For this review, take the finished solid that the model builds, in its own axes (mm). A direction names the side the tool comes from. Give positions to 0.01 mm unless a question says otherwise; leave off trailing zeros. Loops run counter-clockwise (first coordinate to the right, second up) from the corner with the lowest first, then second, coordinate; pieces in that order, holes last. Notation, with made-up numbers: (22.25, 61) - (38.25, 61) arc R22 ccw to (38.25, 93) - close; hole circle Ø9 at (-39, -38.75). An arc over 180 degrees is marked (long way). Put each result on its own line as item: value.
Autodesk Inventor part; units mm, degrees
ref_plane "YZ Plane" through (0, 0, 0) normal (1, 0, 0) x (0, 1, 0)
ref_plane "XZ Plane" through (0, 0, 0) normal (0, 1, 0) x (-1, 0, 0)
ref_plane "XY Plane" through (0, 0, 0) normal (0, 0, 1) x (1, 0, 0)
sketch "Sketch1" plane through (0, 0, 0) normal (0, 1, 0) x (-1, 0, 0)
  arc A0 (7.5, 0) -> (-7.5, 0) centre (0, 0) ccw
  arc A1 (2.4, 0) -> (-2.4, 0) centre (0, 0) ccw
  line L0 (-7.5, 0) -> (7.5, 0) construction
  line L1 (0, 0) -> (0, 11.6178) construction
  line L2 (-7.5, 0) -> (-7.5, -7.5)
  line L3 (-2.4, 0) -> (-2.4, -7.5)
  line L4 (2.4, 0) -> (2.4, -7.5)
  line L5 (7.5, 0) -> (7.5, -7.5)
  line L6 (-7.5, -7.5) -> (-2.4, -7.5)
  line L7 (2.4, -7.5) -> (7.5, -7.5)
  dimension "d0" = 15
  dimension "d2" = 7.5
  dimension "d3" = 4.8
  dimension "d6" = 7.5
  dimension "d8" = 7.5
extrude "Extrusion1" add sketch "Sketch1" against normal blind 3
sketch "Sketch2" plane through (0, -3, 0) normal (0, -1, 0) x (1, 0, 0)
  arc A0 (7.5, 0) -> (-7.5, 0) centre (0, 0) ccw
  line L0 (-7.5, 0) -> (-7.5, -7.5)
  line L1 (-2.4, -7.5) -> (-2.4, 0)
  arc A1 (2.4, 0) -> (-2.4, 0) centre (0, 0) ccw
  line L2 (2.4, 0) -> (2.4, -7.5)
  line L3 (7.5, -7.5) -> (7.5, 0)
  arc A2 (2.4, -5.4991) -> (-2.4, -5.4991) centre (0, 0) ccw
  arc A3 (7.5, 0) -> (-7.5, 0) centre (0, 0) ccw
  line L4 (-7.5, 0) -> (-7.5, -7.5)
  line L5 (-2.4, -7.5) -> (-2.4, -5.4991)
  line L6 (2.4, -5.4991) -> (2.4, -7.5)
  line L7 (7.5, -7.5) -> (7.5, 0)
  line L8 (-7.5, -7.5) -> (-2.4, -7.5)
  line L9 (2.4, -7.5) -> (7.5, -7.5)
  dimension "d11" = 6
extrude "Extrusion2" add sketch "Sketch2" along normal blind 3 contours L3 L9 L2 A2 L1 L8 L0 A0
fillet "Fillet1" radius 1.2 1 edges at (7.5, -3, -7.5)
fillet "Fillet2" radius 1.2 3 edges at (2.4, -3, -7.5) (-2.4, -3, -7.5) (-7.5, -3, -7.5)
sketch "Sketch3" plane through (0, -3, 0) normal (0, -1, 0) x (1, 0, 0)
  arc A0 (2.4, -5.4991) -> (-2.4, -5.4991) centre (0, 0) ccw
  line L0 (-2.4, -5.4991) -> (-2.4, 0)
  arc A1 (2.4, 0) -> (-2.4, 0) centre (0, 0) ccw
  line L1 (2.4, 0) -> (2.4, -5.4991)
  line L2 (0, 13.9059) -> (0, -15.9339) construction
  line L3 (-15.9969, 0.3837) -> (17.7517, -5.5671) construction
  line L4 (-15.1634, 5.1107) -> (18.5852, -0.84) construction
  line L5 (-2.4, -15.573) -> (-2.4, 20.0388) construction
  line L6 (2.4, -5.4991) -> (2.4, -2.8602)
  line L7 (4.9988, -3.3184) -> (2.4, -2.8602)
  line L8 (-4.9988, 3.3184) -> (-2.4, 2.8602)
  line L9 (-2.4, 5.4991) -> (-2.4, 2.8602)
  arc A2 (-3, 5.1962) -> (-4.9988, 3.3184) centre (0, 0) ccw
  arc A3 (2.4, -5.4991) -> (4.9988, -3.3184) centre (0, 0) ccw
  dimension "d27" = 80
extrude "Extrusion3" add sketch "Sketch3" along normal blind 3 contours L1 L7 A0 | L9 L8 A0
equation "\"d0\" = HeadConnectorOuterSize"
equation "\"d2\" = 0.5 * HeadConnectorOuterSize"
equation "\"d3\" = HeadConnectorWidth"
equation "\"d6\" = 0.5 * HeadConnectorOuterSize"
equation "\"d8\" = 0.5 * HeadConnectorOuterSize"
equation "\"d9\" = HeadConnectorOuterHeight"
equation "\"d11\" = 0.5 * HeadConnectorDiam"
equation "\"d12\" = HeadConnectorHeight"
equation "\"d14\" = 0.2 * HeadConnectorProportion"
equation "\"d15\" = 0.2 * HeadConnectorProportion"
equation "\"d28\" = HeadConnectorHeight"
equation "\"HeadConnectorDiam\" = 2 * HeadConnectorProportion"
equation "\"HeadConnectorWidth\" = 0.8 * HeadConnectorProportion"
equation "\"HeadConnectorOuterSize\" = 2.5 * HeadConnectorProportion"
equation "\"HeadConnectorHeight\" = 0.5 * HeadConnectorProportion"
equation "\"HeadConnectorOuterHeight\" = 0.5 * HeadConnectorProportion"
equation "\"HeadConnectorTolerance\" = 0.2"
equation "\"HeadConnectorProportion\" = 0.6"
properties part number "HeadConnector"
1) For faces 1 (the face through (-2.4, -4, 4)), 2 (the face through (-7.158, -3.042, -7.139)), 3 (the face through (-2.761, -3.042, -7.158)), 4 (the face through (-3.718, -4.479, 3.093)), 5 (the face through (5, -3, -7.5)), list the 3-axis set-ups (+Z, -Z, +X, -X, +Y, -Y) from which the entire face can be reached by the end or side of a thin tool; tool diameter is ignored.
Geometry check:
face 1: -Z, -Y
face 2: -Z, -X, +Y, -Y
face 3: -Z, +Y, -Y
face 4: -Y
face 5: -Z, +X, -X, +Y, -Y
2) Insertion check: pin 1 Ø1.5 at (x, y) = (1, -2) entering from +Z; pin 2 Ø1.5 at (x, y) = (3.5, -3) entering from +Z; pin 3 Ø3 at (y, z) = (-5, 4) entering from +X. Each pin has a flat end and moves straight along its axis. Give the tip position at first contact, or say it passes through.
Geometry check:
pin 1: stops at z = 7.5
pin 2: stops at z = 6.98
pin 3: stops at x = 7.07
3) Take a section at A-A on z = -2. State the section outline as (x, y) points.
Geometry check:
outline: (-7.5, -6) - (-5.66, -6) - (-5.66, -3) - (-2.4, -3) - (-2.4, 0) - (-7.5, 0) - close; (2.4, -3) - (5.66, -3) - (5.66, -6) - (7.5, -6) - (7.5, 0) - (2.4, 0) - close
4) Take a section at C-C on y = -2.65. State the section outline as (x, z) points.
Geometry check:
outline: (-7.5, -6.3) arc R1.2 ccw to (-6.3, -7.5) - (-3.6, -7.5) arc R1.2 ccw to (-2.4, -6.3) - (-2.4, 0) arc R2.4 cw to (2.4, 0) - (2.4, -6.3) arc R1.2 ccw to (3.6, -7.5) - (6.3, -7.5) arc R1.2 ccw to (7.5, -6.3) - (7.5, 0) arc R7.5 ccw to (-7.5, 0) - close
5) Take a section at D-D on z = 4.25. State the section outline as (x, y) points.
Geometry check:
outline: (-6.18, -6) - (-2.4, -6) - (-2.4, -3) - (4.24, -3) - (4.24, -6) - (6.18, -6) - (6.18, 0) - (-6.18, 0) - close
6) Draft analysis for pull direction X (two halves, no side actions). For faces 6 (the face through (0, -3, 3)), 7 (the face through (-7.5, -3, -3)), 8 (the face through (2, 0, 2)), state which applies: pulls with the +X half, pulls with the -X half, needs draft (parallel to the pull), parting line crosses it, or undercut.
Geometry check:
face 6: undercut
face 7: pulls with the -X half
face 8: needs draft
7) Take a section at B-B on x = 0. State the section outline as (y, z) points, and give its area (3 significant figures).
Geometry check:
outline: (-6, 6) - (-3, 6) - (-3, 2.4) - (0, 2.4) - (0, 7.5) - (-6, 7.5) - close
area: 19.8 mm²
8) Wall thickness on line 1 (X direction, y = -0.8, z = -5.25); line 2 (Y direction, x = 3.25, z = 1.75); line 3 (X direction, y = -3.9, z = 0): over which ranges is each line inside the solid? List them lowest first.
Geometry check:
line 1: x = -7.5 to -2.4, 2.4 to 7.5
line 2: y = -3 to 0
line 3: x = -7.5 to -6, 6 to 7.5
